For this review, take the finished solid that the model builds, in its own axes (mm). A direction names the side the tool comes from. Round coordinates to 2 decimals unless told otherwise and drop trailing zeros. Order: outer loops, then holes, each group sorted by start corner. A loop starts at its lowest first (then second) coordinate and runs counter-clockwise, first axis right, second up. Notation, with made-up numbers: M 86,57 L 123,57 A10 cw 123,61 Z; hole C 55,36 d9. An arc over 180 degrees is marked long. Answer as a JSON object with one key per item and string values.
from build123d import *

# Parameters (mm, degrees)
SKETCH017_R       = 1.85
EXTRUDE014_DEPTH  = 12
CYLINDER007_R     = 5
CYLINDER007_DEPTH = 1
EXTRUDE013_DEPTH  = 15


with BuildPart() as extrude014:
    # Sketch017 → Extrude014 (new body)
    with BuildSketch(Plane.XZ):
        Polygon((11.75, 36), (11.75, 19), (-17.25, 19), (-23.25, 25), (-23.25, 30), (-17.25, 36), align=None)
        with Locations((-16, 27.481564)):
            Circle(SKETCH017_R, mode=Mode.SUBTRACT)
    extrude(amount=-EXTRUDE014_DEPTH)


with BuildPart() as unprintable:
    # Cylinder007 → Cylinder007 (new body)
    with BuildSketch(Plane(origin=(-16, 18, 27.5), x_dir=(1, 0, 0), z_dir=(0, -1, 0))):
        Circle(CYLINDER007_R)
    extrude(amount=CYLINDER007_DEPTH)


with BuildPart() as body007:
    # Sketch018 → Extrude013 (new body)
    with BuildSketch(Plane.XY.offset(50)):
        with BuildLine():
            ThreePointArc((8.75, 0), (1.006685, 8.691898), (-8.518363, 2))
            Line((-8.518363, 2), (-22.518363, 2))
            Line((-22.518363, 5), (-22.518363, 2))
            Line((-10.633085, 5), (-22.518363, 5))
            ThreePointArc((11.75, 0), (2.561616, 11.467372), (-10.633085, 5))
            Line((8.75, 0), (11.75, 0))
        make_face()
    extrude(amount=EXTRUDE013_DEPTH)


with BuildPart() as body007_1:
    # Extrude013 placement: moved
    add(body007.part.moved(Location((0, 0, -30))))

    # Fusion016: union unprintable
    add(unprintable.part)

    # Common001: intersect Extrude014
    add(extrude014.part, mode=Mode.INTERSECT)


with BuildPart() as part_mirroring008:
    # Part__Mirroring008: instance of Body007
    add(body007_1.part.mirror(Plane(origin=(0, 0, 0), x_dir=(1, 0, 0), z_dir=(0, 1, 0))))


solid = part_mirroring008.part
1) Insertion check: P1, Ø1, axis at x = -5, z = 33, coming from the +Y side; P2, Ø5, axis at x = -17, z = 23.5, coming from the -Y side; P3, Ø2, axis at x = -16, z = 27.48, coming from the +Y side; P4, Ø8, axis at x = -14.5, z = 25, coming from the +Y side. Each pin has a flat end and moves straight along its axis. Give the tip position at first contact, or say it passes through.
Geometry check:
{"P1": "stops at y = -6.81", "P2": "stops at y = -5", "P3": "passes through", "P4": "stops at y = -2"}
2) Add section B-B on x = -16. State the section outline as (y, z) points.
Geometry check:
{"outline": "M -5,20 L -2,20 L -2,25.63 L -5,25.63 Z; M -5,29.33 L -2,29.33 L -2,35 L -5,35 Z"}
3) Add section C-C on z = 26. State the section outline as (x, y) points.
Geometry check:
{"outline": "M -22.52,-5 L -17.11,-5 L -17.11,-2 L -22.52,-2 Z; M -14.89,-5 L -10.63,-5 A11.75 ccw 11.75,0 L 8.75,0 A8.75 cw -8.52,-2 L -14.89,-2 Z"}
4) Add section A-A on y = -7. State the section outline as (x, z) points.
Geometry check:
{"outline": "M -9.44,20 L -5.25,20 L -5.25,35 L -9.44,35 Z; M 5.25,20 L 9.44,20 L 9.44,35 L 5.25,35 Z"}
5) Add section D-D on z = 33.25. State the section outline as (x, y) points, and give its area (3 significant figures).
Geometry check:
{"outline": "M -20,-5 L -10.63,-5 A11.75 ccw 11.75,0 L 8.75,0 A8.75 cw -8.52,-2 L -20,-2 Z", "area": "117 mm²"}
6) Mouldability with a two-part tool opening along Z and no side actions: class faces 3 (the flat face through (-2, -9, 35)), 4 (the flat face through (-20.35, -3.48, 22.1)), 5 (the cylindrical face through (-15.15, -3.48, 25.84)), 6 (the flat face through (-14, -5, 27)) as +Z half, -Z half, draft (parallel to the pull), parting line (faces both ways), or undercut.
Geometry check:
{"face 3": "+Z half", "face 4": "-Z half", "face 5": "undercut", "face 6": "draft"}
7) For L1, parallel to Z at x = -16, y = -2.75; L2, parallel to Y at x = -19, z = 31.5; L3, parallel to Y at x = 0, z = 31.5, list the stretches that pass through material, from the lowest coordinate up.
Geometry check:
{"L1": "z = 20 to 25.63, 29.33 to 35", "L2": "y = -5 to -2", "L3": "y = -11.75 to -8.75"}
8) Machinability: for faces 1 (the flat face through (-2, -9, 20)), 2 (the flat face through (-14, -2, 27)), which of the approach directions +Z, -Z, +X, -X, +Y, -Y give a long, thin tool a straight path to every point of the face, cutting with its end or side? Answer none if there is none.
Geometry check:
{"face 1": "-Z, +X, -X, +Y, -Y", "face 2": "+Z, -Z, -X, +Y"}
